Design review of the part built by this model. Coordinates are the model's own, in mm. Face numbers are marked on the shaded views. A direction names the side the tool comes from. Give positions to 0.01 mm unless a question says otherwise; leave off trailing zeros. Write each loop counter-clockwise with the first axis right and the second up, starting at its lowest first coordinate (ties: lowest second). Pieces come first, ordered by that corner, then holes.
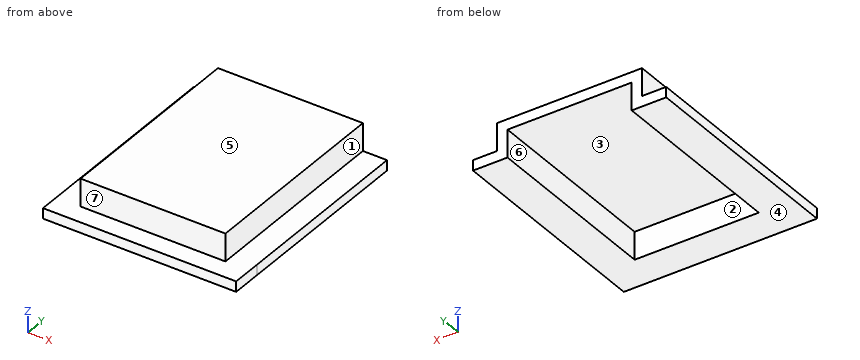
```python
from build123d import *

# Parameters (mm, degrees)
SKETCH1_W           = 42
SKETCH1_H           = 58
BOSS_EXTRUDE1_DEPTH = 3
SKETCH2_W           = 3
SKETCH2_H           = 58
BOSS_EXTRUDE2_DEPTH = 8
SKETCH3_W           = 3
SKETCH3_H           = 58
BOSS_EXTRUDE3_DEPTH = 8
SKETCH4_W           = 36.040635574
SKETCH4_H           = 4.348824295
BOSS_EXTRUDE4_DEPTH = 8
SKETCH5_W           = 10
SKETCH5_H           = 53.666567446
BOSS_EXTRUDE5_DEPTH = 3
SKETCH6_W           = 10
SKETCH6_H           = 54.883518579
BOSS_EXTRUDE6_DEPTH = 3
SKETCH7_W           = 55.997152208
SKETCH7_H           = 10
BOSS_EXTRUDE7_DEPTH = 3


with BuildPart() as part:
    # Sketch1 → Boss-Extrude1 (new body)
    with BuildSketch(Plane.XY):
        with Locations((0, -1.5)):
            Rectangle(SKETCH1_W, SKETCH1_H)
    extrude(amount=BOSS_EXTRUDE1_DEPTH)

    # Sketch2 → Boss-Extrude2 (add)
    with BuildSketch(Plane(origin=(0, 0, 0), x_dir=(-1, 0, 0), z_dir=(0, 0, -1))):
        with Locations((-19.5, -1.5)):
            Rectangle(SKETCH2_W, SKETCH2_H)
    extrude(amount=BOSS_EXTRUDE2_DEPTH)

    # Sketch3 → Boss-Extrude3 (add)
    with BuildSketch(Plane(origin=(0, 0, 0), x_dir=(-1, 0, 0), z_dir=(0, 0, -1))):
        with Locations((19.5, -1.5)):
            Rectangle(SKETCH3_W, SKETCH3_H)
    extrude(amount=BOSS_EXTRUDE3_DEPTH)

    # Sketch4 → Boss-Extrude4 (add)
    with BuildSketch(Plane(origin=(0, 0, 0), x_dir=(-1, 0, 0), z_dir=(0, 0, -1))):
        with Locations((0.020317787, -28.325587852)):
            Rectangle(SKETCH4_W, SKETCH4_H)
    extrude(amount=BOSS_EXTRUDE4_DEPTH)

    # Sketch5 → Boss-Extrude5 (add)
    with BuildSketch(Plane(origin=(0, 0, -8), x_dir=(-1, 0, 0), z_dir=(0, 0, -1))):
        with Locations((23, 0.666716277)):
            Rectangle(SKETCH5_W, SKETCH5_H)
    extrude(amount=-BOSS_EXTRUDE5_DEPTH)

    # Sketch6 → Boss-Extrude6 (add)
    with BuildSketch(Plane(origin=(0, 0, -8), x_dir=(-1, 0, 0), z_dir=(0, 0, -1))):
        with Locations((-23, 0.05824071)):
            Rectangle(SKETCH6_W, SKETCH6_H)
    extrude(amount=-BOSS_EXTRUDE6_DEPTH)

    # Sketch7 → Boss-Extrude7 (add)
    with BuildSketch(Plane(origin=(0, 0, -8), x_dir=(-1, 0, 0), z_dir=(0, 0, -1))):
        with Locations((0.001423896, -31.166567446)):
            Rectangle(SKETCH7_W, SKETCH7_H)
    extrude(amount=-BOSS_EXTRUDE7_DEPTH)


solid = part.part
```
(1) Consider section D-D, the plane x = 25. Give the boundary of the cut face in (y, z), then the cut area to 3 significant figures.
Resolved:
outline: (-36.17, -8) - (27.5, -8) - (27.5, -5) - (-36.17, -5) - close
area: 191 mm2
(2) Consider section C-C, the plane z = 1.5. Give the boundary of the cut face in (x, y), then the cut area to 3 significant figures.
Resolved:
outline: (-21, -30.5) - (21, -30.5) - (21, 27.5) - (-21, 27.5) - close
area: 2,440 mm2
(3) Clearance check with flat-ended pins moving along their axes: P1, Ø4, axis at y = 4.5, z = -4.5, coming from the +X side; P2, Ø1.5, axis at x = 10, z = -5, coming from the +Y side. State where each tip first meets the part, or that it passes through.
Resolved:
P1: stops at x = 28
P2: stops at y = -26.15
(4) Mouldability with a two-part tool opening along X and no side actions: class the marked faces 1, 2, 3 and 4 as pulls with the +X half, pulls with the -X half, needs draft (parallel to the pull), parting line crosses it, or undercut.
Resolved:
face 1: pulls with the +X half
face 2: undercut
face 3: undercut
face 4: needs draft
(5) Tool access review of the marked faces 5, 6 and 7: name each direction out of +Z, -Z, +X, -X, +Y, -Y from which nothing blocks a thin tool from reaching the whole face with its end or side.
Resolved:
face 5: +Z, +X, -X, +Y, -Y
face 6: -Z, +Y
face 7: +Z, +X, -X, -Y
(6) To check wall thickness, follow L1, parallel to X at y = -3, z = -3.25; L2, parallel to X at y = -10.5, z = -6.25; L3, parallel to X at y = -7.5, z = 0.75. State the ranges of each line that lie inside material, in increasing order.
Resolved:
L1: x = -21 to -18, 18 to 21
L2: x = -28 to -18, 18 to 28
L3: x = -21 to 21
(7) Consider section B-B, the plane x = 13. Give the boundary of the cut face in (y, z).
Resolved:
outline: (-36.17, -8) - (-26.15, -8) - (-26.15, 0) - (27.5, 0) - (27.5, 3) - (-30.5, 3) - (-30.5, -5) - (-36.17, -5) - close
(8) Consider section A-A, the plane y = 10. Give the boundary of the cut face in (x, z), then the cut area to 3 significant figures.
Resolved:
outline: (-28, -8) - (-18, -8) - (-18, 0) - (18, 0) - (18, -8) - (28, -8) - (28, -5) - (21, -5) - (21, 3) - (-21, 3) - (-21, -5) - (-28, -5) - close
area: 216 mm2
